Source: CAD feature listing. Evaluate the final solid. Frame: model axes, mm. A direction names the side the tool comes from. Give positions to 0.01 mm unless a question says otherwise; leave off trailing zeros. Write each loop counter-clockwise with the first axis right and the second up, starting at its lowest first coordinate (ties: lowest second). Pieces come first, ordered by that corner, then holes. Notation, with made-up numbers: M -30.75,34.25 L 4.25,34.25 A34 cw 4.25,64.25 Z; hole C -24.75,-0.5 d6. An arc over 180 degrees is marked long. Return JSON: item names as keys, results as strings.
```python
from build123d import *

# Parameters (mm, degrees)
SKETCH1_W           = 42.57
SKETCH1_H           = 20
BOSS_EXTRUDE1_DEPTH = 100
SKETCH2_W           = 37.57
SKETCH2_H           = 15
CUT_EXTRUDE1_DEPTH  = 111.508845347
CUT_EXTRUDE2_DEPTH  = 111.508845347


with BuildPart() as part:
    # Sketch1 → Boss-Extrude1 (new body)
    with BuildSketch(Plane(origin=(0, 0, 0), x_dir=(0, 0, -1), z_dir=(1, 0, 0))):
        with Locations((21.285, 10)):
            Rectangle(SKETCH1_W, SKETCH1_H)
    extrude(amount=BOSS_EXTRUDE1_DEPTH)

    # Sketch2 → Cut-Extrude1 (cut, through all)
    with BuildSketch(Plane.ZY):
        with Locations((-21.285, 10)):
            Rectangle(SKETCH2_W, SKETCH2_H)
    extrude(amount=-CUT_EXTRUDE1_DEPTH, mode=Mode.SUBTRACT)

    # Sketch3 → Cut-Extrude2 (cut, through all)
    with BuildSketch(Plane.XY):
        Polygon((0, 0), (34.641016151, 20), (0, 20), align=None)
        Polygon((100, 20), (65.358983849, 0), (100, 0), align=None)
    extrude(amount=-CUT_EXTRUDE2_DEPTH, mode=Mode.SUBTRACT)


solid = part.part
```
1) Line query: line 1 (Z direction, x = 33, y = 13); line 2 (Y direction, x = 37.5, z = -27); line 3 (Y direction, x = 85, z = -10). Output: solid intervals per line, ascending. Write a range as [from, to].
Numbers:
{"line 1": "z = [-42.57, -40.07], [-2.5, 0]", "line 2": "y = [0, 2.5], [17.5, 20]", "line 3": "y = [17.5, 20]"}
2) Contact query for a flat-ended pin moving along its axis: pin 1 Ø3 at (x, z) = (67.5, -21.5) entering from -Y. Output: stop coordinate, or through.
Numbers:
{"pin 1": "stops at y = 0.37"}
3) Cut plane D-D, the plane x = 71. Return the cut outline in (y, z), then the cut area to 3 significant figures.
Numbers:
{"outline": "M 3.26,-42.57 L 20,-42.57 L 20,0 L 3.26,0 L 3.26,-2.5 L 17.5,-2.5 L 17.5,-40.07 L 3.26,-40.07 Z", "area": "178 mm²"}
4) Draft query along Y for faces 1 (the face through (49, 10, -2.5)), 2 (the face through (49, 10, -42.57)), 3 (the face through (32, 0, -21)), 4 (the face through (37, 2.5, -22)). Return one class per face: released by +Y, released by -Y, zero draft, split by the parting line, or undercut.
Numbers:
{"face 1": "undercut", "face 2": "zero draft", "face 3": "released by -Y", "face 4": "undercut"}
5) Cut plane A-A, the plane z = -33. Return the cut outline in (x, y).
Numbers:
{"outline": "M 0,0 L 65.36,0 L 69.69,2.5 L 4.33,2.5 Z; M 30.31,17.5 L 95.67,17.5 L 100,20 L 34.64,20 Z"}
6) Set-up query: faces 5 (the face through (3.127, 1.805, -22.762)), 6 (the face through (63, 17.5, -22)). Return all of +Z, -Z, +X, -X, +Y, -Y with unobstructed straight access to the full face (end or side cutting, diameter ignored); none if empty.
Numbers:
{"face 5": "+Z, -Z, -X, +Y", "face 6": "+X, -X"}
7) Cut plane C-C, the plane y = 8.5. Return the cut outline in (x, z).
Numbers:
{"outline": "M 14.72,-42.57 L 80.08,-42.57 L 80.08,-40.07 L 14.72,-40.07 Z; M 14.72,-2.5 L 80.08,-2.5 L 80.08,0 L 14.72,0 Z"}
8) Cut plane B-B, the plane x = 57.5. Return the cut outline in (y, z), then the cut area to 3 significant figures.
Numbers:
{"outline": "M 0,-42.57 L 20,-42.57 L 20,0 L 0,0 Z; hole M 2.5,-40.07 L 17.5,-40.07 L 17.5,-2.5 L 2.5,-2.5 Z", "area": "288 mm²"}
